Input: part model. Units: mm. Frame: model coordinates. A direction names the side the tool comes from. Coordinates: 2 decimals unless noted, no trailing zeros. Write each loop counter-clockwise with the first axis right and the second up, starting at its lowest first coordinate (ties: lowest second). Pieces come first, ordered by that corner, then holes. Notation, with made-up numbers: (34.5, -5) - (55.5, -5) arc R18 ccw to (55.5, 26) - close; hole circle Ø8 at (44.25, 65.25). An arc over 180 degrees is marked (long way). One line per question, with ' | ' between items. Start each with the question number.
1) First-contact query: P1, Ø1.5, axis at y = -0.5, z = -1.5, coming from the +X side; P2, Ø1, axis at y = -3.5, z = 0.5, coming from the -X side; P3, Ø6, axis at y = 3.5, z = 3, coming from the -X side. Flat tips, straight axial feed; report the tip coordinate or a pass-through.
2) Section query A-A on z = 8. Return loops of the section in (x, y).
3) Reachability of faces 1 (the flat face through (0, 0, 29.5)), 2 (the cylindrical face through (-2.43, 0.77, -9.15)) from +Z, -Z, +X, -X, +Y, -Y: full face, straight path, thin tool, end or side. Return the list, or none.
4) Line query: line 1 (Y direction, x = 2, z = 6); line 2 (X direction, y = -1.25, z = 16.5); line 3 (Y direction, x = -6, z = 2.5). Output: solid intervals per line, ascending.
```python
from build123d import *

# Parameters (mm, degrees)
SKETCH1_R           = 7.5
BOSS_EXTRUDE1_DEPTH = 29.5
SKETCH2_R           = 2.55
BOSS_EXTRUDE2_DEPTH = 10
FILLET1_R           = 0.7
FILLET2_R           = 10


with BuildPart() as part:
    # Sketch1 → Boss-Extrude1 (new body)
    with BuildSketch(Plane.XY):
        with Locations(Location((0, 0, 0), (0, 0, 180))):
            Circle(SKETCH1_R)
    extrude(amount=BOSS_EXTRUDE1_DEPTH)

    # Sketch2 → Boss-Extrude2 (add)
    with BuildSketch(Plane(origin=(0, 0, 0), x_dir=(-1, 0, 0), z_dir=(0, 0, -1))):
        Circle(SKETCH2_R)
    extrude(amount=BOSS_EXTRUDE2_DEPTH)

    # Fillet1
    fillet1_edges = [part.edges().sort_by_distance(p)[0] for p in [
        (7.5, 0, 0),
        (7.5, 0, 29.5),
    ]]
    fillet(fillet1_edges, radius=FILLET1_R)

    # Fillet2
    fillet2_edges = [part.edges().sort_by_distance(p)[0] for p in [
        (2.55, 0, 0),
    ]]
    fillet(fillet2_edges, radius=FILLET2_R - 0.0001)  # a hair under: the kernel refuses the full size


solid = part.part
```
Answer key:
1) P1: x = 6 | P2: x = -6.86 | P3: x = -7.48
2) outline: circle Ø15 at (0, 0)
3) face 1: +Z, +X, -X, +Y, -Y | face 2: -Z
4) line 1: -7.23 to 7.23 | line 2: -7.4 to 7.4 | line 3: -4.5 to 4.5
